Work out the finished part from the listing and answer in its coordinate system (mm). A direction names the side the tool comes from. Round coordinates to 2 decimals unless told otherwise and drop trailing zeros. Order: outer loops, then holes, each group sorted by start corner. A loop starts at its lowest first (then second) coordinate and runs counter-clockwise, first axis right, second up. Notation, with made-up numbers: (10, 71) - (51, 71) arc R34 cw to (51, 109) - close; hole circle Ø6 at (30.25, 8). An arc over 180 degrees is marked (long way). One line per question, with ' | ' between items. Start each with the question number.
from build123d import *

# Parameters (mm, degrees)
SKETCH_1_R               = 13
EXTRUDE_1_DEPTH          = 3.7
SKETCH_2_W               = 2
SKETCH_2_H               = 4.2
SKETCH_2_W_2             = 4.2
SKETCH_2_H_2             = 2
EXTRUDE_2_DEPTH          = 7.9
SKETCH_3_R               = 2.4
SKETCH_3_R_2             = 0.5
EXTRUDE_3_DEPTH          = 7.9
PATTERN_CIRCULAR_1_COUNT = 6


with BuildPart() as part:
    # 草图1 → 凸台-拉伸1 (new body)
    with BuildSketch(Plane.XY):
        Circle(SKETCH_1_R)
    extrude(amount=EXTRUDE_1_DEPTH)

    # 草图2 → 凸台-拉伸2 (add)
    with BuildSketch(Plane.XY.offset(3.7)):
        Rectangle(SKETCH_2_W, SKETCH_2_H)
        Rectangle(SKETCH_2_W_2, SKETCH_2_H_2)
    extrude(amount=EXTRUDE_2_DEPTH)

    # 草图3 → 凸台-拉伸3 (add)
    with BuildSketch(Plane.XY.offset(3.7)):
        with Locations((-5.656854249, 5.656854249)):
            Circle(SKETCH_3_R)
        with Locations((-5.656854249, 5.656854249)):
            Circle(SKETCH_3_R_2, mode=Mode.SUBTRACT)
    extrude_3 = extrude(amount=EXTRUDE_3_DEPTH)

    # 阵列(圆周)1: 凸台-拉伸3 ×6 about axis
    pattern_circular_1_axis = Axis((0, 0, 0), (0, 0, 1))
    for i in range(1, PATTERN_CIRCULAR_1_COUNT):
        add(extrude_3.rotate(pattern_circular_1_axis, i * 360 / PATTERN_CIRCULAR_1_COUNT))


solid = part.part
1) Determine the mould class of faces 6 (the flat face through (2, 7, 11.6)), 7 (the cylindrical face through (-0.78, -5.704, 7.595)), 8 (the flat face through (1, -1.6, 7.6)) for opening direction X: released by +X, released by -X, zero draft, split by the parting line, or undercut.
2) For faces 1 (the cylindrical face through (2.179, 8.216, 7.595)), 2 (the flat face through (0, 2.1, 8)), 3 (the flat face through (0, -2.1, 8)), 4 (the flat face through (-2.1, 0, 8)), 5 (the flat face through (-1.6, 1, 7.6)), determine the directions among +Z, -Z, +X, -X, +Y, -Y from which every point of the face is accessible in a straight line to the end or side of a thin tool.
3) Section C-C on y = -4 is taken. Give the vertices of the cut face in (x, z), and give its area (3 significant figures).
4) Flat-ended cylindrical pins translate along their axes: pin 1 (1.5 mm diameter, centred on x = 5.5, z = 3, fed in from -Y); pin 2 (4 mm diameter, centred on y = 7, z = 10, fed in from +X); pin 3 (1 mm diameter, centred on x = 3, z = 7.5, fed in from -Y). Find the tip coordinate at first contact, or state that the pin passes through.
5) Section B-B on x = 8.75 is taken. Give the vertices of the cut face in (y, z).
6) Section D-D on z = 1 is taken. Give the vertices of the cut face in (x, y), and give its area (3 significant figures).
7) Section A-A on z = 7.75 is taken. Give the number of separate pieces and of enclosed holes in the cut face, and give its area (3 significant figures).
8) Straight lines are drawn through the part: line 1 (X direction, y = -7.5, z = 9.25); line 2 (Z direction, x = -4.5, y = -6.5); line 3 (X direction, y = -1.75, z = 8.5). For each, find the intervals that lie inside material, in ascending order.
Recorded:
1) face 6: zero draft | face 7: undercut | face 8: released by +X
2) face 1: +Z | face 2: +Z, -X | face 3: +Z, +X | face 4: +Z, +Y | face 5: +Z, -X, +Y
3) outline: (-12.37, 0) - (12.37, 0) - (12.37, 3.7) - (7.39, 3.7) - (7.39, 11.6) - (3.92, 11.6) - (3.92, 3.7) - (-6.3, 3.7) - (-6.3, 11.6) - (-9.15, 11.6) - (-9.15, 3.7) - (-12.37, 3.7) - close | area: 142 mm²
4) pin 1: stops at y = -12.1 | pin 2: stops at x = 4.47 | pin 3: stops at y = -6.71
5) outline: (-9.61, 0) - (9.61, 0) - (9.61, 3.7) - (4.24, 3.7) - (4.24, 11.6) - (-0.1, 11.6) - (-0.1, 3.7) - (-9.61, 3.7) - close
6) outline: circle Ø26 at (0, 0) | area: 531 mm²
7) separate pieces: 7 | enclosed holes: 6 | area: 117 mm²
8) line 1: x = -4.46 to -2.52, -1.63 to 0.32, 4.12 to 7.19 | line 2: z = 0 to 3.7 | line 3: x = -10.11 to -8.11, -7.34 to -5.35, -1 to 1
